Design review of the part built by this model. Coordinates are the model's own, in mm. Round coordinates to 2 decimals unless told otherwise and drop trailing zeros. Loops run counter-clockwise (first coordinate to the right, second up) from the corner with the lowest first, then second, coordinate; pieces in that order, holes last. Notation, with made-up numbers: M 65,88.5 L 110,88.5 A18 ccw 110,110.5 Z; hole C 71.25,19.5 d2. An arc over 180 degrees is marked long. Answer as CSV lines item,"result". Start each with the question number.
from build123d import *

# Parameters (mm, degrees)
F0_W     = 1219.2
F0_H     = 914.4
F1_DEPTH = 914.4
F2_SIZE  = 254
F3_R     = 12.7


with BuildPart() as f1:
    # F0 (on Top) → F1 (new body)
    with BuildSketch(Plane.XY):
        Rectangle(F0_W, F0_H)
    extrude(amount=F1_DEPTH)

    # F2
    f2_edges = [f1.edges().sort_by_distance(p)[0] for p in [
        (0, -457.2, 914.4),
    ]]
    chamfer(f2_edges, length=F2_SIZE)

    # F3
    f3_edges = [f1.edges().sort_by_distance(p)[0] for p in [
        (609.6, 127, 914.4),
        (609.6, -330.2, 787.4),
        (609.6, -457.2, 330.2),
        (-609.6, -457.2, 330.2),
        (-609.6, -330.2, 787.4),
        (-609.6, 127, 914.4),
    ]]
    fillet(f3_edges, radius=F3_R)


solid = f1.part
Item 1: Consider section A-A, the plane x = 282. Write out the cut boundary in (y, z), then the cut area to 3 significant figures.
Item 2: To check wall thickness, follow line 1 (Y direction, x = 373.5, z = 704.5); line 2 (Y direction, x = 351, z = 755); line 3 (Z direction, x = 521.5, y = -379.5). State the ranges of each line that lie inside material, in increasing order.
Item 3: Insertion check: pin 1 Ø3 at (x, y) = (356.5, -255.5) entering from +Z. The pin has a flat end and moves straight along its axis. Give the tip position at first contact, or say it passes through.
Found:
1,outline,"M -457.2,0 L 457.2,0 L 457.2,914.4 L -203.2,914.4 L -457.2,660.4 Z"
1,area,"804,000 mm^2"
2,line 1,"y = -413.1 to 457.2"
2,line 2,"y = -362.6 to 457.2"
2,line 3,"z = 0 to 738.1"
3,pin 1,"stops at z = 863.6"
